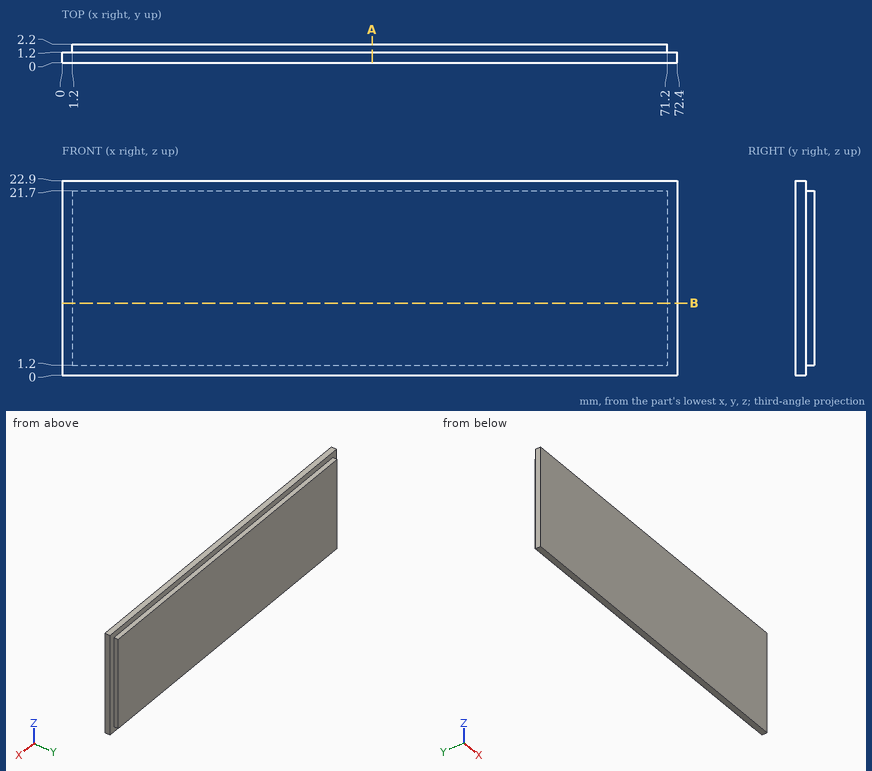
Geometry check sheet. Reference: drawing and pictorial views, mm from the part's lowest x, y, z. Coordinates: 2 decimals unless noted, no trailing zeros. Order: outer loops, then holes, each group sorted by start corner. A loop starts at its lowest first (then second) coordinate and runs counter-clockwise, first axis right, second up. Notation, with made-up numbers: (63.25, 23) - (113.25, 23) arc R20 ccw to (113.25, 54) - close; hole circle Ø9 at (51, 52.25). An arc over 180 degrees is marked (long way). Answer in a Markdown table with one row per item. Add a question column.
1) Material ranges on line 1 along X through (y, z) = (1.35, 20.75); line 2 along Z through (x, y) = (22, 2.05), recorded low to high. Write a range as [from, to].
2) Cross-section at B-B, the plane z = 8.5. Record the cut outline in (x, y), then the cut area to 3 significant figures.
3) Cross-section at A-A, the plane x = 36.5. Record the cut outline in (y, z).
Check result:
| question | item | result |
|---|---|---|
| 1 | line 1 | x = [1.2, 71.2] |
| 1 | line 2 | z = [1.2, 21.7] |
| 2 | outline | (0, 0) - (72.4, 0) - (72.4, 1.2) - (71.2, 1.2) - (71.2, 2.2) - (1.2, 2.2) - (1.2, 1.2) - (0, 1.2) - close |
| 2 | area | 157 mm² |
| 3 | outline | (0, 0) - (1.2, 0) - (1.2, 1.2) - (2.2, 1.2) - (2.2, 21.7) - (1.2, 21.7) - (1.2, 22.9) - (0, 22.9) - close |
